The figure shows three views and two pictorial views of one solid part (mm, origin at its lowest corner). Answer the questions. A direction names the side the tool comes from. Coordinates: 2 decimals unless noted, no trailing zeros. Order: outer loops, then holes, each group sorted by start corner. A loop starts at its lowest first (then second) coordinate and runs counter-clockwise, first axis right, second up. Notation, with made-up numbers: (47, -4) - (106, -4) arc R15 cw to (106, 6) - close; hole circle Ø3 at (80, 0). An arc over 180 degrees is marked (long way). Answer as a JSON object with one key per item and string values. Group by question number.
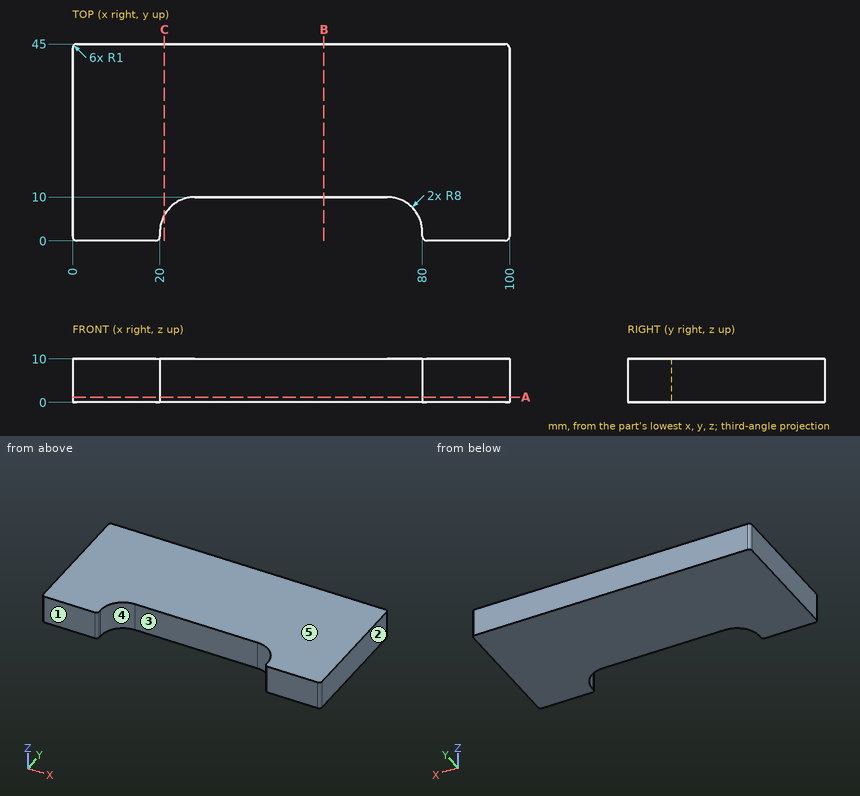
1. For the marked faces 4 and 5, determine the directions among +Z, -Z, +X, -X, +Y, -Y from which every point of the face is accessible in a straight line to the end or side of a thin tool.
2. For a pull along X with two mould halves and no side action, classify the marked faces 1, 2 and 3 as pulls with the +X half, pulls with the -X half, needs draft (parallel to the pull), parting line crosses it, or undercut.
3. A cutting plane is placed at C-C on x = 21. Write down the section's boundary in (y, z).
4. A cutting plane is placed at A-A on z = 1.25. Write down the section's boundary in (x, y).
5. Straight lines are drawn through the part: L1, parallel to X at y = 7, z = 7.5 (3 decimals); L2, parallel to Y at x = 52.5, z = 4.5; L3, parallel to X at y = 6, z = 8.75. For each, find the intervals that lie inside material, in ascending order.
6. A cutting plane is placed at B-B on x = 57.5. Write down the section's boundary in (y, z), and give its area (3 significant figures).
7. Given pin 1 (5 mm diameter, centred on x = 24.5, z = 6.5, fed in from -Y), flat-ended and moving along its own axis, determine where the tip first touches the part or whether it passes through.
Derived:
{
 "1": {"face 4": "+Z, -Z, -Y", "face 5": "+Z, +X, -X, +Y, -Y"},
 "2": {"face 1": "needs draft", "face 2": "pulls with the +X half", "face 3": "undercut"},
 "3": {"outline": "(5.87, 0) - (45, 0) - (45, 10) - (5.87, 10) - close"},
 "4": {"outline": "(0, 1) arc R1 ccw to (1, 0) - (19, 0) arc R1 ccw to (20, 1) - (20, 2) arc R8 cw to (28, 10) - (72, 10) arc R8 cw to (80, 2) - (80, 1) arc R1 ccw to (81, 0) - (99, 0) arc R1 ccw to (100, 1) - (100, 44) arc R1 ccw to (99, 45) - (1, 45) arc R1 ccw to (0, 44) - close"},
 "5": {"L1": "x = 0 to 21.755, 78.245 to 100", "L2": "y = 10 to 45", "L3": "x = 0 to 21.07, 78.93 to 100"},
 "6": {"outline": "(10, 0) - (45, 0) - (45, 10) - (10, 10) - close", "area": "350 mm2"},
 "7": {"pin 1": "stops at y = 7.29"}
}
